Check sheet for the modelled part. Datum: model origin and axes. Units: mm. A direction names the side the tool comes from. Round coordinates to 2 decimals unless told otherwise and drop trailing zeros. Loops run counter-clockwise (first coordinate to the right, second up) from the corner with the lowest first, then second, coordinate; pieces in that order, holes last. Notation, with made-up numbers: (-21.5, -35) -> (13.5, -35) arc R31 ccw to (13.5, -2) -> close; hole circle Ø3 at (-28.5, 63). An arc over 180 degrees is marked (long way). One line per item, written item: value. Start each with the question number.
1. Go/stop test with flat-tipped pins: pin 1 (3 mm diameter, centred on x = -0.5, z = 34, fed in from -Y); pin 2 (1.5 mm diameter, centred on x = -6.5, z = 16.5, fed in from -Y); pin 3 (3 mm diameter, centred on y = 6, z = 37, fed in from -X). Record where each tip stops, or that it passes through.
2. Material ranges on L1, parallel to Z at x = -2, y = -8; L2, parallel to X at y = 3, z = 37.5; L3, parallel to Z at x = -9.5, y = 9, recorded low to high.
3. Cross-section at B-B on x = -5.5. Record the cut outline in (y, z).
4. Cross-section at C-C on y = -16.5. Record the cut outline in (x, z), then the cut area to 3 significant figures.
5. Cross-section at D-D on x = 1. Record the cut outline in (y, z), then the cut area to 3 significant figures.
6. Set-up check for faces 1 (the face through (6.733, 7, 35)), 2 (the face through (-16.6, 5, 8)): record each of +Z, -Z, +X, -X, +Y, -Y from which the full face is reachable in a straight line by a thin tool's end or side.
7. Cross-section at A-A on z = 19. Record the cut outline in (x, y), then the cut area to 3 significant figures.
from build123d import *

# Parameters (mm, degrees)
F0_W     = 40
F0_H     = 40
F1_DEPTH = 30
F3_DEPTH = 20
F5_DEPTH = 10
F7_DEPTH = 10
F8_ANGLE = 90


with BuildPart() as f1:
    # F0 (on Top) → F1 (new body)
    with BuildSketch(Plane.XY):
        Rectangle(F0_W, F0_H)
    extrude(amount=F1_DEPTH)

    # F2 (on face) → F3 (cut)
    with BuildSketch(Plane.YZ.offset(20)):
        Polygon((20, 30), (-20, 30), (-20, 0), (-10, 0), (20, 20), align=None)
    extrude(amount=-F3_DEPTH, mode=Mode.SUBTRACT)

    # F4 (on face) → F5 (cut)
    with BuildSketch(Plane.YZ):
        Polygon((10, 30), (-20, 30), (-20, 10), (-10, 20), (10, 20), align=None)
    extrude(amount=-F5_DEPTH, mode=Mode.SUBTRACT)

    # F6 (on face) → F7 (cut)
    with BuildSketch(Plane.YZ.offset(20)):
        Polygon((15, 6.666667), (15, 16.666667), (0, 6.666667), align=None)
    extrude(amount=-F7_DEPTH, mode=Mode.SUBTRACT)


with BuildPart() as f1_1:
    # F8: moved
    add(f1.part.rotate(Axis((-20, 0, 0), (0, -1, 0)), F8_ANGLE))


with BuildPart() as f1_2:
    # F9: moved
    add(f1_1.part.moved(Location((33.4, 0, 0))))


solid = f1_2.part
Taken from the geometry:
1. pin 1: stops at y = 15
1. pin 2: stops at y = -10.85
1. pin 3: stops at x = 6.73
2. L1: z = 0 to 20
2. L2: x = 6.73 to 13.4
2. L3: z = 0 to 10
3. outline: (-20, 0) -> (20, 0) -> (20, 40) -> (18.35, 40) -> (18.35, 20) -> (-11.1, 20) -> (-11.1, 10) -> (-20, 10) -> close
4. outline: (-16.6, 0) -> (13.4, 0) -> (13.4, 20) -> (-0.1, 20) -> (-0.1, 10) -> (-16.6, 10) -> close
4. area: 435 mm2
5. outline: (-20, 0) -> (20, 0) -> (20, 40) -> (15, 40) -> (15, 30) -> (8.6, 30) -> (8.6, 20) -> (-17.6, 20) -> (-17.6, 10) -> (-20, 10) -> close
5. area: 940 mm2
6. face 1: +Z, -X, -Y
6. face 2: +Z, -Z, -X, +Y, -Y
7. outline: (-16.6, 10) -> (-6.6, 10) -> (-6.6, -10) -> (3.4, -20) -> (13.4, -20) -> (13.4, 20) -> (-16.6, 20) -> close
7. area: 850 mm2
